Part model, mm, in its own coordinate system. Round coordinates to 2 decimals unless told otherwise and drop trailing zeros. Write each loop counter-clockwise with the first axis right and the second up, starting at its lowest first coordinate (ties: lowest second). Pieces come first, ordered by that corner, then holes.
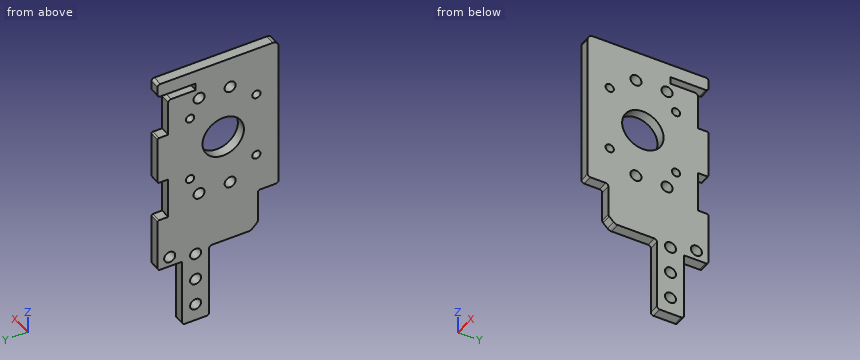
```python
from build123d import *

# Parameters (mm, degrees)
SKETCH6_R                   = 9.525
SKETCH6_R_2                 = 1.905
SKETCH6_R_3                 = 2.5527
SIDE_PLATE_EXTRUDE_DEPTH    = 4.7498
SKETCH15_R                  = 2.5527
CUSTOM_NUTSTRIP_HOLES_DEPTH = 5.7498
SKETCH43_W                  = 3.175
SKETCH43_H                  = 12.7
CUT_EXTRUDE19_DEPTH         = 5.7498
SKETCH73_W                  = 15.875
SKETCH73_H                  = 4.7625
SKETCH73_W_2                = 22.733
SKETCH73_W_3                = 6.35
BOSS_EXTRUDE28_DEPTH        = 4.7498
SKETCH108_W                 = 9.525
SKETCH108_H                 = 11.1125
SKETCH108_R                 = 2.5527
BOSS_EXTRUDE35_DEPTH        = 4.7498
SKETCH90_W                  = 18.959213894
SKETCH90_H                  = 4.8895
SKETCH90_W_2                = 34.925
SKETCH90_H_2                = 31.877
SIDE_PLATE_TOLERENCES_DEPTH = 5.7498
CHAMFER8_SIZE               = 12.7
FILLET15_R                  = 2.54
FILLET26_R                  = 1.27
FILLET29_R                  = 0.635
SKETCH109_W                 = 19.05
SKETCH109_H                 = 9.525
CUT_EXTRUDE20_DEPTH         = 5.7498
FILLET30_R                  = 1.27


with BuildPart() as part:
    # Sketch6 → Side Plate Extrude (new body)
    with BuildSketch(Plane.ZY.offset(104.775)):
        Polygon((162.052, -25.4), (162.052, 25.4), (77.649686106, 25.4), (77.649686106, 19.05), (36.374686106, 19.05), (36.374686106, 6.35), (71.299686106, 6.35), (71.299686106, -25.4), align=None)
        with Locations((123.825, 0)):
            Circle(SKETCH6_R, mode=Mode.SUBTRACT)
        with Locations((108.585, -15.24)):
            Circle(SKETCH6_R_2, mode=Mode.SUBTRACT)
        with Locations((108.585, 15.24)):
            Circle(SKETCH6_R_2, mode=Mode.SUBTRACT)
        with Locations((139.065, 15.24)):
            Circle(SKETCH6_R_2, mode=Mode.SUBTRACT)
        with Locations((139.065, -15.24)):
            Circle(SKETCH6_R_2, mode=Mode.SUBTRACT)
        with Locations((147.7645, 11.1125)):
            Circle(SKETCH6_R_3, mode=Mode.SUBTRACT)
        with Locations((99.6315, 11.1125)):
            Circle(SKETCH6_R_3, mode=Mode.SUBTRACT)
        with Locations((99.6315, -3.175)):
            Circle(SKETCH6_R_3, mode=Mode.SUBTRACT)
        with Locations((147.7645, -3.175)):
            Circle(SKETCH6_R_3, mode=Mode.SUBTRACT)
    extrude(amount=SIDE_PLATE_EXTRUDE_DEPTH)

    # Sketch15 → Custom Nutstrip Holes (cut, through all)
    with BuildSketch(Plane.ZY.offset(109.5248)):
        with Locations((44.312186106, 12.7)):
            Circle(SKETCH15_R)
        with Locations((57.012186106, 12.7)):
            Circle(SKETCH15_R)
        with Locations((69.712186106, 12.7)):
            Circle(SKETCH15_R)
    extrude(amount=-CUSTOM_NUTSTRIP_HOLES_DEPTH, mode=Mode.SUBTRACT)

    # Sketch43 → Cut-Extrude19 (cut, through all)
    with BuildSketch(Plane.ZY.offset(109.5248)):
        with Locations((154.1145, 19.05)):
            Rectangle(SKETCH43_W, SKETCH43_H)
    extrude(amount=-CUT_EXTRUDE19_DEPTH, mode=Mode.SUBTRACT)

    # Sketch73 → Boss-Extrude28 (add, through all)
    with BuildSketch(Plane.ZY.offset(109.5248)):
        with Locations((85.587186106, 27.78125)):
            Rectangle(SKETCH73_W, SKETCH73_H)
        with Locations((123.698, 27.78125)):
            Rectangle(SKETCH73_W_2, SKETCH73_H)
        with Locations((158.877, 27.78125)):
            Rectangle(SKETCH73_W_3, SKETCH73_H)
    extrude(amount=-BOSS_EXTRUDE28_DEPTH)

    # Sketch108 → Boss-Extrude35 (add, through all)
    with BuildSketch(Plane(origin=(-104.775, 0, 0), x_dir=(0, 0, -1), z_dir=(1, 0, 0))):
        with Locations((-72.887186106, 24.60625)):
            Rectangle(SKETCH108_W, SKETCH108_H)
        with Locations((-72.887186106, 24.60625)):
            Circle(SKETCH108_R, mode=Mode.SUBTRACT)
    extrude(amount=-BOSS_EXTRUDE35_DEPTH)

    # Sketch90 → Side Plate Tolerences (cut, through all)
    with BuildSketch(Plane(origin=(-104.775, 0, 0), x_dir=(0, 0, -1), z_dir=(1, 0, 0))):
        Polygon((-152.4508, 12.7), (-155.7782, 12.7), (-155.7782, 30.1625), (-152.4508, 30.1625), (-134.9883, 30.1625), (-134.9883, 25.273), (-152.4508, 25.273), align=None)
        with Locations((-102.928093053, 27.71775)):
            Rectangle(SKETCH90_W, SKETCH90_H)
        Polygon((-68.124686106, 19.05), (-36.374686106, 19.05), (-36.374686106, 18.923), (-68.124686106, 18.923), (-68.251686106, 18.923), (-68.251686106, 30.1625), (-68.124686106, 30.1625), align=None)
        with Locations((-53.837186106, -9.4615)):
            Rectangle(SKETCH90_W_2, SKETCH90_H_2)
    extrude(amount=-SIDE_PLATE_TOLERENCES_DEPTH, mode=Mode.SUBTRACT)

    # Chamfer8
    chamfer8_edges = [part.edges().sort_by_distance(p)[0] for p in [
        (-107.1499, -25.4, 71.299686106),
    ]]
    chamfer(chamfer8_edges, length=CHAMFER8_SIZE)

    # Fillet15
    fillet15_edges = [part.edges().sort_by_distance(p)[0] for p in [
        (-107.1499, -25.4, 162.052),
        (-107.1499, -25.4, 83.999686106),
        (-107.1499, -12.7, 71.299686106),
    ]]
    fillet(fillet15_edges, radius=FILLET15_R)

    # Fillet26
    fillet26_edges = [part.edges().sort_by_distance(p)[0] for p in [
        (-107.1499, 30.1625, 162.052),
        (-107.1499, 30.1625, 155.7782),
        (-107.1499, 25.273, 152.4508),
        (-107.1499, 18.923, 36.374686106),
        (-107.1499, 30.1625, 68.251686106),
        (-107.1499, 6.477, 36.374686106),
        (-107.1499, 6.477, 71.299686106),
    ]]
    fillet(fillet26_edges, radius=FILLET26_R)

    # Fillet29
    fillet29_edges = [part.edges().sort_by_distance(p)[0] for p in [
        (-107.1499, 30.1625, 134.9883),
        (-107.1499, 30.1625, 112.4077),
        (-107.1499, 30.1625, 93.448486106),
    ]]
    fillet(fillet29_edges, radius=FILLET29_R)

    # Sketch109 → Cut-Extrude20 (cut, through all)
    with BuildSketch(Plane(origin=(-104.775, 0, 0), x_dir=(0, 0, -1), z_dir=(1, 0, 0))):
        with Locations((-80.824686106, -20.6375)):
            Rectangle(SKETCH109_W, SKETCH109_H)
    extrude(amount=-CUT_EXTRUDE20_DEPTH, mode=Mode.SUBTRACT)

    # Fillet30
    fillet30_edges = [part.edges().sort_by_distance(p)[0] for p in [
        (-107.1499, -15.875, 74.474686106),
        (-107.1499, -25.4, 90.349686106),
        (-107.1499, -15.875, 90.349686106),
    ]]
    fillet(fillet30_edges, radius=FILLET30_R)


solid = part.part
```
Q1. Cut at C-C on y = 3.5. Write the cut outline in (x, z) (3 decimals), plus the area to 3 significant figures.
Values follow:
outline: (-109.525, 71.3) - (-104.775, 71.3) - (-104.775, 114.966) - (-109.525, 114.966) - close; (-109.525, 132.684) - (-104.775, 132.684) - (-104.775, 162.052) - (-109.525, 162.052) - close
area: 347 mm2
Q2. Wall check: L1, parallel to Y at x = -107.25, z = 71.5; L2, parallel to Y at x = -105.6, z = 57; L3, parallel to Y at x = -105.4, z = 78 (1 decimal). Give the ranges that are in metal, low to high.
Values follow:
L1: y = -12.64 to 10.88, 14.52 to 22.46, 26.75 to 30.16
L2: y = 6.48 to 10.15, 15.25 to 18.92
L3: y = -15.9 to 30.2
Q3. Drop flat-ended pins along their axis: pin 1 (4 mm diameter, centred on y = -3.18, z = 99.63, fed in from +X); pin 2 (1.5 mm diameter, centred on x = -105.5, z = 96.5, fed in from +Y); pin 3 (2.5 mm diameter, centred on x = -108, z = 79.5, fed in from -Y) (3 decimals); pin 4 (1.7 mm diameter, centred on x = -108, z = 153.5, fed in from +Y). Give the stop position or say it passes through.
Values follow:
pin 1: passes through
pin 2: stops at y = 25.27
pin 3: stops at y = -15.875
pin 4: stops at y = 12.7
Q4. Cut at A-A on y = -8. Write the cut outline in (x, z) (3 decimals), plus the area to 3 significant figures.
Values follow:
outline: (-109.525, 71.3) - (-104.775, 71.3) - (-104.775, 118.655) - (-109.525, 118.655) - close; (-109.525, 128.995) - (-104.775, 128.995) - (-104.775, 162.052) - (-109.525, 162.052) - close
area: 382 mm2
Q5. Cut at B-B on x = -106.1. State how many separate pieces and enclosed holes the cut face has, plus the area to 3 significant figures.
Values follow:
separate pieces: 1
enclosed holes: 13
area: 4,590 mm2
